Work out the finished part from the listing and answer in its coordinate system (mm). A direction names the side the tool comes from. Give positions to 0.01 mm unless a question says otherwise; leave off trailing zeros. Order: outer loops, then holes, each group sorted by start corner. A loop starts at its lowest first (then second) coordinate and runs counter-clockwise, first axis right, second up.
```python
from build123d import *

# Parameters (mm, degrees)
SKETCH1_W            = 20.5
SKETCH1_H            = 9
BOSS_EXTRUDE1_DEPTH  = 6
SKETCH2_W            = 25
SKETCH2_H            = 58
BOSS_EXTRUDE2_DEPTH  = 5
LPATTERN1_COUNT      = 2
LPATTERN1_PITCH      = 49
LPATTERN2_COUNT      = 2
LPATTERN2_PITCH      = 25.5
CUT_EXTRUDE1_REACH   = 62.632
SKETCH3_R            = 2
LPATTERN3_COUNT      = 2
LPATTERN3_PITCH      = 10.3
LPATTERN3_COUNT_DIR2 = 2
LPATTERN3_PITCH_DIR2 = 49
SKETCH8_W            = 25
SKETCH8_H            = 50
BOSS_EXTRUDE3_DEPTH  = 6
LPATTERN4_COUNT      = 2
LPATTERN4_PITCH      = 36.5
M6_CLEARANCE_HOLE1_D = 6.6
CHAMFER2_SIZE        = 10
LPATTERN5_COUNT      = 2
LPATTERN5_PITCH      = 20
FILLET1_R            = 10


with BuildPart() as part:
    # Sketch1 → Boss-Extrude1 (new body)
    with BuildSketch(Plane.XY):
        with Locations((10.25, 4.5)):
            Rectangle(SKETCH1_W, SKETCH1_H)
    boss_extrude1 = extrude(amount=BOSS_EXTRUDE1_DEPTH)

    # Sketch2 → Boss-Extrude2 (add)
    with BuildSketch(Plane(origin=(20.5, 0, 0), x_dir=(0, 0, -1), z_dir=(1, 0, 0))):
        with Locations((6.5, -20)):
            Rectangle(SKETCH2_W, SKETCH2_H)
    boss_extrude2 = extrude(amount=BOSS_EXTRUDE2_DEPTH)

    # LPattern1: Boss-Extrude1 ×2
    with Locations(*[(0, -i * LPATTERN1_PITCH, 0) for i in range(1, LPATTERN1_COUNT)]):
        add(boss_extrude1)

    # LPattern2: Boss-Extrude2 ×2
    with Locations(*[(-i * LPATTERN2_PITCH, 0, 0) for i in range(1, LPATTERN2_COUNT)]):
        add(boss_extrude2)

    # Sketch3 → Cut-Extrude1 (cut, up to next)
    with BuildSketch(Plane.XY.offset(6), mode=Mode.PRIVATE) as cut_extrude1_sk1:
        with Locations((5.1, 4.5)):
            Circle(SKETCH3_R)
    cut_extrude1_tool1 = extrude(cut_extrude1_sk1.sketch, amount=-CUT_EXTRUDE1_REACH, mode=Mode.PRIVATE) & part.part
    cut_extrude1 = cut_extrude1_tool1.solids().sort_by_distance((5.1, 4.5, 6))[0]
    add(cut_extrude1, mode=Mode.SUBTRACT)

    # LPattern3: Cut-Extrude1 2 × 2
    with Locations(*[(i * LPATTERN3_PITCH, -j * LPATTERN3_PITCH_DIR2, 0) for i in range(LPATTERN3_COUNT) for j in range(LPATTERN3_COUNT_DIR2) if (i, j) != (0, 0)]):
        add(cut_extrude1, mode=Mode.SUBTRACT)

    # Sketch8 → Boss-Extrude3 (add)
    with BuildSketch(Plane(origin=(25.5, 0, 0), x_dir=(0, 0, -1), z_dir=(1, 0, 0))):
        with Locations((6.5, 27.997404855)):
            Rectangle(SKETCH8_W, SKETCH8_H)
    boss_extrude3 = extrude(amount=BOSS_EXTRUDE3_DEPTH)

    # LPattern4: Boss-Extrude3 ×2
    with Locations(*[(-i * LPATTERN4_PITCH, 0, 0) for i in range(1, LPATTERN4_COUNT)]):
        add(boss_extrude3)

    # M6 Clearance Hole1 (through all)
    with Locations(Plane.ZY.offset(11)):
        with Locations((-6.5, 21)):
            m6_clearance_hole1 = Hole(M6_CLEARANCE_HOLE1_D / 2)

    # Chamfer2
    # the kernel refuses this chamfer: 10 mm, written as the material it adds along each edge
    with BuildSketch(Plane(origin=(-5, 2.997404855, 6), x_dir=(-0.9996219169112968, 0.027495876610586403, 0), z_dir=(0, 0, -1))) as chamfer2_piece_1_section:
        Polygon((CHAMFER2_SIZE * 0.999621916911, -CHAMFER2_SIZE * 0.0274958766106), (-CHAMFER2_SIZE * 0.0274958766106, -CHAMFER2_SIZE * 0.999621916911), (0, 0), align=None)
    chamfer2_piece_1 = extrude(amount=25, mode=Mode.PRIVATE)
    chamfer2_piece_1 = split(chamfer2_piece_1, bisect_by=Plane(origin=(-11, -0.75268974, -6.5), z_dir=(1, 0, 0)), keep=Keep.TOP, mode=Mode.PRIVATE)
    add(chamfer2_piece_1)
    with BuildSketch(Plane(origin=(25.5, 2.997404855, 6), x_dir=(-0.02749587661058666, -0.9996219169112968, 0), z_dir=(0, 0, -1))) as chamfer2_piece_2_section:
        Polygon((CHAMFER2_SIZE * 0.999621916911, -CHAMFER2_SIZE * 0.0274958766106), (-CHAMFER2_SIZE * 0.0274958766106, -CHAMFER2_SIZE * 0.999621916911), (0, 0), align=None)
    chamfer2_piece_2 = extrude(amount=25, mode=Mode.PRIVATE)
    chamfer2_piece_2 = split(chamfer2_piece_2, bisect_by=Plane(origin=(31.5, -0.75268974, -6.5), z_dir=(-1, 0, 0)), keep=Keep.TOP, mode=Mode.PRIVATE)
    add(chamfer2_piece_2)

    # LPattern5: M6 Clearance Hole1 ×2
    with Locations(*[(0, i * LPATTERN5_PITCH, 0) for i in range(1, LPATTERN5_COUNT)]):
        add(m6_clearance_hole1, mode=Mode.SUBTRACT)

    # Fillet1
    fillet1_edges = [part.edges().sort_by_distance(p)[0] for p in [
        (28.5, 52.997404855, 6),
        (28.5, 52.997404855, -19),
        (-8, 52.997404855, 6),
        (-8, 52.997404855, -19),
    ]]
    fillet(fillet1_edges, radius=FILLET1_R)


solid = part.part
```
1. Which of the six approach directions +Z, -Z, +X, -X, +Y, -Y give full straight-line access (tool end or side, diameter ignored) to faces 5 (the face through (10, -44, 0)), 6 (the face through (10, 0, 3)), 7 (the face through (7, 9, 2)), 8 (the face through (31.5, 26, -6))?
Findings below:
face 5: -Z, +Y, -Y
face 6: +Z, -Z
face 7: +Z, -Z, +Y
face 8: +Z, -Z, +X, +Y, -Y
2. The part is cut by section C-C (x = 5.1). Write down the section's boundary in (y, z).
Findings below:
outline: (-49, 0) - (-46.5, 0) - (-46.5, 6) - (-49, 6) - close; (-42.5, 0) - (-40, 0) - (-40, 6) - (-42.5, 6) - close; (0, 0) - (2.5, 0) - (2.5, 6) - (0, 6) - close; (6.5, 0) - (9, 0) - (9, 6) - (6.5, 6) - close
3. Straight lines are drawn through the part: probe 1 along Y at (x, z) = (15.4, 3.8); probe 2 along X at (y, z) = (34.5, 4); probe 3 along Y at (x, z) = (-7.85, -6.5). For each, find the intervals that lie inside material, in ascending order.
Findings below:
probe 1: y = -49 to -46.5, -42.5 to -40, 0 to 2.5, 6.5 to 9
probe 2: x = -11 to -5, 25.5 to 31.5
probe 3: y = -4.15 to 17.7, 24.3 to 37.7, 44.3 to 53
4. Given P1, Ø12.5, axis at x = 3.5, z = -9, coming from the +Y side; P2, Ø5, axis at x = 15.4, y = 4.5, coming from the -Z side; P3, Ø3.5, axis at x = 5.1, y = 4.5, coming from the +Z side; P4, Ø8, axis at y = -7.5, z = -13, coming from the -X side, each flat-ended and moving along its own axis, determine where each tip first touches the part or whether it passes through.
Findings below:
P1: stops at y = 9
P2: stops at z = 0
P3: passes through
P4: stops at x = -8.5
5. The part is cut by section A-A (y = 41). Write down the section's boundary in (x, z), then the cut area to 3 significant figures.
Findings below:
outline: (-11, -19) - (-5, -19) - (-5, -9.8) - (-11, -9.8) - close; (-11, -3.2) - (-5, -3.2) - (-5, 6) - (-11, 6) - close; (25.5, -19) - (31.5, -19) - (31.5, -9.8) - (25.5, -9.8) - close; (25.5, -3.2) - (31.5, -3.2) - (31.5, 6) - (25.5, 6) - close
area: 221 mm2
6. The part is cut by section B-B (z = -6.5). State how many separate pieces and enclosed holes the cut face has, then the cut area to 3 significant figures.
Findings below:
separate pieces: 6
enclosed holes: 0
area: 1,110 mm2
7. The mould has two halves that part along X. Classify faces 1 (the face through (6.947, 3.734, 3.042)), 2 (the face through (-8, -4, -6)), 3 (the face through (10, 5, 0)), 4 (the face through (7, -49, 2)): pulls with the +X half, pulls with the -X half, needs draft (parallel to the pull), parting line crosses it, or undercut.
Findings below:
face 1: undercut
face 2: pulls with the -X half
face 3: undercut
face 4: needs draft
8. The part is cut by section D-D (y = -17). Write down the section's boundary in (x, z), then the cut area to 3 significant figures.
Findings below:
outline: (-5, -19) - (0, -19) - (0, 6) - (-5, 6) - close; (20.5, -19) - (25.5, -19) - (25.5, 6) - (20.5, 6) - close
area: 250 mm2
